from build123d import *

# Parameters (mm, degrees)
F0_W     = 30
F0_H     = 30
F1_DEPTH = 35
F2_R     = 11.75
F3_DEPTH = 29
F4_W     = 28
F4_H     = 5
F5_DEPTH = 14


with BuildPart() as f1:
    # F0 (on Top) → F1 (new body)
    with BuildSketch(Plane.XY):
        with Locations((13.941668, -72.72828)):
            Rectangle(F0_W, F0_H)
    extrude(amount=F1_DEPTH)

    # F2 (on face) → F3 (cut)
    with BuildSketch(Plane.XY.offset(35)):
        with Locations((13.941668, -72.72828)):
            Circle(F2_R)
    extrude(amount=-F3_DEPTH, mode=Mode.SUBTRACT)

    # F4 (on face) → F5 (cut)
    with BuildSketch(Plane.XZ.offset(87.72828)):
        with Locations((14, 4.5)):
            Rectangle(F4_W, F4_H)
    extrude(amount=-F5_DEPTH, mode=Mode.SUBTRACT)


solid = f1.part
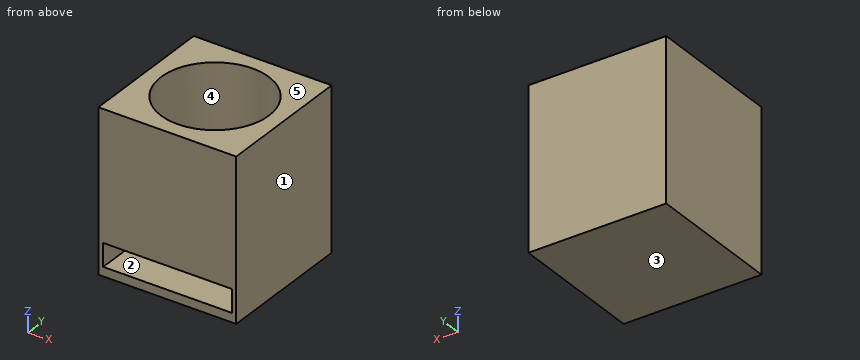
Part model, mm, in its own coordinate system. Face numbers are marked on the shaded views. A direction names the side the tool comes from. Round coordinates to 2 decimals unless told otherwise and drop trailing zeros. Write each loop counter-clockwise with the first axis right and the second up, starting at its lowest first coordinate (ties: lowest second). Pieces come first, ordered by that corner, then holes. Notation, with made-up numbers: M 5,29.5 L 62,29.5 A21 cw 62,55.5 Z; hole C 84,3.5 d6. An arc over 180 degrees is marked long. Return JSON: item names as keys, results as strings. Group by question number.
(1) Which spindle directions (+Z, -Z, +X, -X, +Y, -Y) get a long thin tool onto all of the face, cutting with end or side? Do the marked faces 4 and 5. Say none if no direction does.
(2) Saw through at C-C on z = 19. Write the cut outline in (x, y).
(3) Two-plate mould, pull along Z, no slides. Class the marked faces 1, 2 and 3: +Z half, -Z half, draft (parallel to the pull), parting line (faces both ways), or undercut.
(4) Pin check, flat tips, straight feed: pin 1 Ø7 at (x, y) = (13, -80.5) entering from -Z; pin 2 Ø1.5 at (x, z) = (17, 4) entering from -Y; pin 3 Ø7 at (x, y) = (16, -80) entering from +Z; pin 4 Ø6 at (x, y) = (22.5, -73.5) entering from +Z. Stop position of each tip, or through.
(5) Saw through at B-B on y = -77. Write the cut outline in (x, z).
(6) Drill centre lines: probe 1 along X at (y, z) = (-81.25, 4); probe 2 along Z at (x, y) = (25.75, -82); probe 3 along Y at (x, z) = (4, 19). Where is each one in solid material? Low to high.
(7) Saw through at A-A on x = 3. Write the cut outline in (y, z).
(8) Saw through at D-D on x = 20.5. Write the cut outline in (y, z), then the cut area to 3 significant figures.
Returned:
{
 "1": {"face 4": "+Z", "face 5": "+Z, +X, -X, +Y, -Y"},
 "2": {"outline": "M -1.06,-87.73 L 28.94,-87.73 L 28.94,-57.73 L -1.06,-57.73 Z; hole C 13.94,-72.73 d23.5"},
 "3": {"face 1": "draft", "face 2": "undercut", "face 3": "-Z half"},
 "4": {"pin 1": "z = 0", "pin 2": "y = -73.73", "pin 3": "z = 2", "pin 4": "z = 6"},
 "5": {"outline": "M -1.06,0 L 28.94,0 L 28.94,35 L 24.89,35 L 24.89,7 L 28,7 L 28,2 L 0,2 L 0,7 L 3,7 L 3,35 L -1.06,35 Z"},
 "6": {"probe 1": "-1.06 to 0, 28 to 28.94", "probe 2": "0 to 2, 7 to 35", "probe 3": "-87.73 to -78.99, -66.47 to -57.73"},
 "7": {"outline": "M -87.73,0 L -57.73,0 L -57.73,35 L -68.45,35 L -68.45,6 L -73.73,6 L -73.73,2 L -87.73,2 Z; M -87.73,7 L -77.01,7 L -77.01,35 L -87.73,35 Z"},
 "8": {"outline": "M -87.73,0 L -57.73,0 L -57.73,35 L -62.98,35 L -62.98,6 L -73.73,6 L -73.73,2 L -87.73,2 Z; M -87.73,7 L -82.48,7 L -82.48,35 L -87.73,35 Z", "area": "423 mm²"}
}
